Source: CAD feature listing. Evaluate the final solid. Frame: model axes, mm. Coordinates: 2 decimals unless noted, no trailing zeros. Write each loop counter-clockwise with the first axis right and the second up, starting at its lowest first coordinate (ties: lowest second). Pieces come first, ordered by that corner, then holes. Notation, with made-up numbers: (25, -39.5) - (53, -39.5) arc R14 ccw to (53, -15.5) - close; hole circle Ø11 at (-11.75, 16.25). An arc over 180 degrees is marked (long way). One line per item, written item: value.
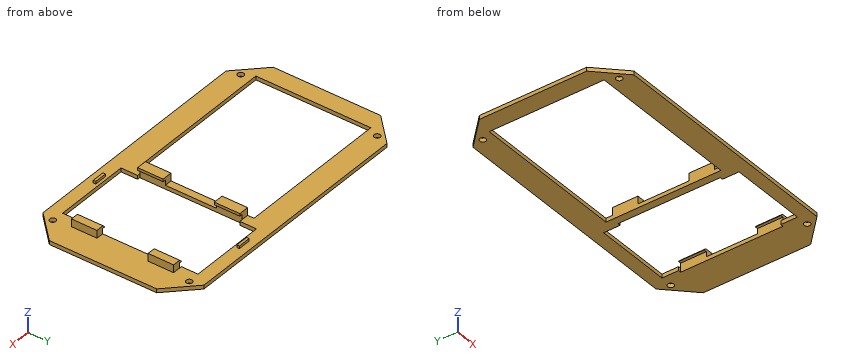
from build123d import *

# Parameters (mm, degrees)
SKETCH_R        = 1.2
PAD_DEPTH       = 1.5
SKETCH001_W     = 60
SKETCH001_H     = 45
SKETCH001_W_2   = 30
SKETCH001_H_2   = 53
POCKET_DEPTH    = 5
SKETCH002_W     = 4
SKETCH002_H     = 10
PAD001_DEPTH    = 3
SKETCH003_W     = 32.2
SKETCH003_H     = 40
POCKET001_DEPTH = 3.5
SKETCH004_W     = 5
SKETCH004_H     = 1
PAD002_DEPTH    = 1
CHAMFER_SIZE    = 0.9


with BuildPart() as pad:
    # Sketch → Pad (new body)
    with BuildSketch(Plane.XY):
        Polygon((-47, 31.5), (47, 31.5), (57.5, 21), (57.5, -21), (47, -31.5), (-47, -31.5), (-57.5, -21), (-57.5, 21), align=None)
        with Locations((-48.25, 26.7)):
            Circle(SKETCH_R, mode=Mode.SUBTRACT)
        with Locations((48.25, 26.7)):
            Circle(SKETCH_R, mode=Mode.SUBTRACT)
        with Locations((-48.25, -26.7)):
            Circle(SKETCH_R, mode=Mode.SUBTRACT)
        with Locations((48.25, -26.7)):
            Circle(SKETCH_R, mode=Mode.SUBTRACT)
    extrude(amount=PAD_DEPTH)


with BuildPart() as pocket:
    # Pocket base: copy of Pad
    add(pad.part)

    # Sketch001 → Pocket (cut)
    with BuildSketch(Plane.XY.offset(1.5)):
        with Locations((-20.5, 0)):
            Rectangle(SKETCH001_W, SKETCH001_H)
        with Locations((28.5, 0)):
            Rectangle(SKETCH001_W_2, SKETCH001_H_2)
    extrude(amount=-POCKET_DEPTH, mode=Mode.SUBTRACT)


with BuildPart() as common:
    # Common base: copy of Pad
    add(pad.part)

    # Common: intersect Pocket
    add(pocket.part, mode=Mode.INTERSECT)


with BuildPart() as fusion:
    # Pad001 base: copy of Common
    add(common.part)

    # Sketch002 → Pad001 (new body)
    with BuildSketch(Plane.XY.offset(1.5)):
        with Locations((11.5, 15)):
            Rectangle(SKETCH002_W, SKETCH002_H)
        with Locations((11.5, -15)):
            Rectangle(SKETCH002_W, SKETCH002_H)
        with Locations((45.5, 15)):
            Rectangle(SKETCH002_W, SKETCH002_H)
        with Locations((45.5, -15)):
            Rectangle(SKETCH002_W, SKETCH002_H)
    extrude(amount=PAD001_DEPTH)

    # Fusion: union Common
    add(common.part)


with BuildPart() as pocket001:
    # Pocket001 base: copy of Fusion
    add(fusion.part)

    # Sketch003 → Pocket001 (cut)
    with BuildSketch(Plane(origin=(0, 0, 0), x_dir=(1, 0, 0), z_dir=(0, 0, -1))):
        with Locations((28.5, 0)):
            Rectangle(SKETCH003_W, SKETCH003_H)
    extrude(amount=-POCKET001_DEPTH, mode=Mode.SUBTRACT)


with BuildPart() as common001:
    # Common001 base: copy of Fusion
    add(fusion.part)

    # Common001: intersect Pocket001
    add(pocket001.part, mode=Mode.INTERSECT)


with BuildPart() as chamfer_body:
    # Pad002 base: copy of Common001
    add(common001.part)

    # Sketch004 → Pad002 (new body)
    with BuildSketch(Plane.XY.offset(1.5)):
        with Locations((22.5, 28.1)):
            Rectangle(SKETCH004_W, SKETCH004_H)
        with Locations((22.5, -28.1)):
            Rectangle(SKETCH004_W, SKETCH004_H)
    extrude(amount=PAD002_DEPTH)

    # Fusion001: union Common001
    add(common001.part)

    # Chamfer
    chamfer_edges = [chamfer_body.edges().sort_by_distance(p)[0] for p in [
        (43.5, -15, 4.5),
        (43.5, 15, 4.5),
    ]]
    chamfer(chamfer_edges, length=CHAMFER_SIZE)


solid = chamfer_body.part
1) Material intervals for line 1 (X direction, y = 13, z = 1.15); line 2 (Y direction, x = -48.25, z = 0.6); line 3 (Y direction, x = -42, z = 1), sorted ascending.
Values found:
line 1: -57.5 to -50.5, 9.5 to 12.4, 44.6 to 57.5
line 2: -30.25 to -27.9, -25.5 to -22.5, 22.5 to 25.5, 27.9 to 30.25
line 3: -31.5 to -22.5, 22.5 to 31.5
2) Section query B-B on y = -24. Output: boundary loops of the cut face in (x, z).
Values found:
outline: (-54.5, 0) - (13.5, 0) - (13.5, 1.5) - (-54.5, 1.5) - close; (43.5, 0) - (54.5, 0) - (54.5, 1.5) - (43.5, 1.5) - close
3) Section query A-A on x = -34. Output: boundary loops of the cut face in (y, z), then the cut area to 3 significant figures.
Values found:
outline: (-31.5, 0) - (-22.5, 0) - (-22.5, 1.5) - (-31.5, 1.5) - close; (22.5, 0) - (31.5, 0) - (31.5, 1.5) - (22.5, 1.5) - close
area: 27.0 mm2
4) Section query C-C on y = -16. Output: boundary loops of the cut face in (x, z), then the cut area to 3 significant figures.
Values found:
outline: (-57.5, 0) - (-50.5, 0) - (-50.5, 1.5) - (-57.5, 1.5) - close; (9.5, 0) - (12.4, 0) - (12.4, 3.5) - (13.5, 3.5) - (13.5, 4.5) - (9.5, 4.5) - close; (43.5, 3.5) - (44.6, 3.5) - (44.6, 0) - (57.5, 0) - (57.5, 1.5) - (47.5, 1.5) - (47.5, 4.5) - (44.4, 4.5) - (43.5, 3.6) - close
area: 53.4 mm2
5) Section query D-D on x = -48.25. Output: boundary loops of the cut face in (y, z).
Values found:
outline: (-30.25, 0) - (-27.9, 0) - (-27.9, 1.5) - (-30.25, 1.5) - close; (-25.5, 0) - (-22.5, 0) - (-22.5, 1.5) - (-25.5, 1.5) - close; (22.5, 0) - (25.5, 0) - (25.5, 1.5) - (22.5, 1.5) - close; (27.9, 0) - (30.25, 0) - (30.25, 1.5) - (27.9, 1.5) - close
6) Contact query for flat-ended pins moving along their axis: P1, Ø1.6, axis at y = -22.5, z = 1, coming from the +X side; P2, Ø1.5, axis at x = -40, y = 24, coming from the +Z side; P3, Ø0.9, axis at y = -14, z = 3, coming from the +X side. Output: stop coordinate, or through.
Values found:
P1: x = 56.8
P2: z = 1.5
P3: x = 47.5
